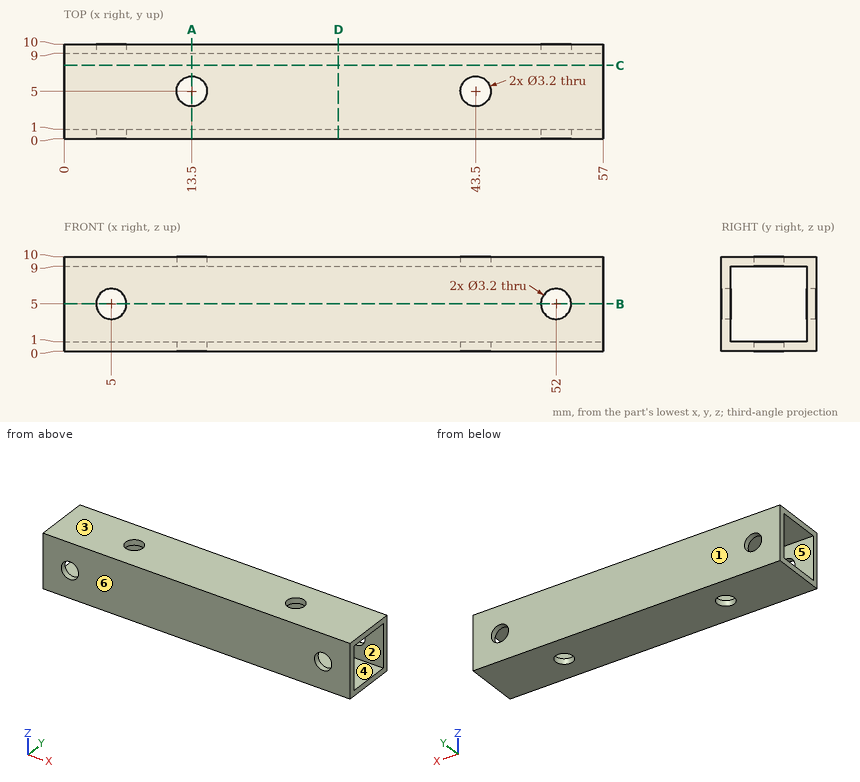
Job drawing, mm, ordinate dimensions from the low corner. One solid piece. A direction names the side the tool comes from. Round coordinates to 2 decimals unless told otherwise and drop trailing zeros. Order: outer loops, then holes, each group sorted by start corner. A loop starts at its lowest first (then second) coordinate and runs counter-clockwise, first axis right, second up. Notation, with made-up numbers: (21, 8) -> (53, 8) arc R31 cw to (53, 36) -> close; hole circle Ø10 at (52, 24.25). An arc over 180 degrees is marked (long way). Answer in a Markdown table with one row per item.
1) Mould opens along Y. For the marked faces 1, 2, 3 and 4 say: released by +Y, released by -Y, zero draft, split by the parting line, or undercut.
Values:
| item | result |
|---|---|
| face 1 | released by +Y |
| face 2 | undercut |
| face 3 | zero draft |
| face 4 | undercut |
2) Band-saw the part on A-A on x = 13.5. Give the cut face in (y, z).
Values:
| item | result |
|---|---|
| outline | (0, 0) -> (3.4, 0) -> (3.4, 1) -> (1, 1) -> (1, 9) -> (3.4, 9) -> (3.4, 10) -> (0, 10) -> close; (6.6, 0) -> (10, 0) -> (10, 10) -> (6.6, 10) -> (6.6, 9) -> (9, 9) -> (9, 1) -> (6.6, 1) -> close |
3) Band-saw the part on B-B on z = 5. Give the cut face in (x, y).
Values:
| item | result |
|---|---|
| outline | (0, 0) -> (3.4, 0) -> (3.4, 1) -> (0, 1) -> close; (0, 9) -> (3.4, 9) -> (3.4, 10) -> (0, 10) -> close; (6.6, 0) -> (50.4, 0) -> (50.4, 1) -> (6.6, 1) -> close; (6.6, 9) -> (50.4, 9) -> (50.4, 10) -> (6.6, 10) -> close; (53.6, 0) -> (57, 0) -> (57, 1) -> (53.6, 1) -> close; (53.6, 9) -> (57, 9) -> (57, 10) -> (53.6, 10) -> close |
4) Band-saw the part on C-C on y = 7.75. Give the cut face in (x, z).
Values:
| item | result |
|---|---|
| outline | (0, 0) -> (57, 0) -> (57, 1) -> (0, 1) -> close; (0, 9) -> (57, 9) -> (57, 10) -> (0, 10) -> close |
5) Wall check: L1, parallel to Y at x = 31.5, z = 5.75; L2, parallel to Z at x = 52, y = 9.55; L3, parallel to X at y = 5, z = 0.35. Give the ranges that are in metal, low to high.
Values:
| item | result |
|---|---|
| L1 | 0 to 1, 9 to 10 |
| L2 | 0 to 3.4, 6.6 to 10 |
| L3 | 0 to 11.9, 15.1 to 41.9, 45.1 to 57 |
6) Band-saw the part on D-D on x = 29. Give the cut face in (y, z), and give its area (3 significant figures).
Values:
| item | result |
|---|---|
| outline | (0, 0) -> (10, 0) -> (10, 10) -> (0, 10) -> close; hole (1, 1) -> (9, 1) -> (9, 9) -> (1, 9) -> close |
| area | 36.0 mm2 |
7) Which spindle directions (+Z, -Z, +X, -X, +Y, -Y) get a long thin tool onto all of the face, cutting with end or side? Do the marked faces 5 and 6. Say none if no direction does.
Values:
| item | result |
|---|---|
| face 5 | +X, -X |
| face 6 | +Z, -Z, +X, -X, -Y |
